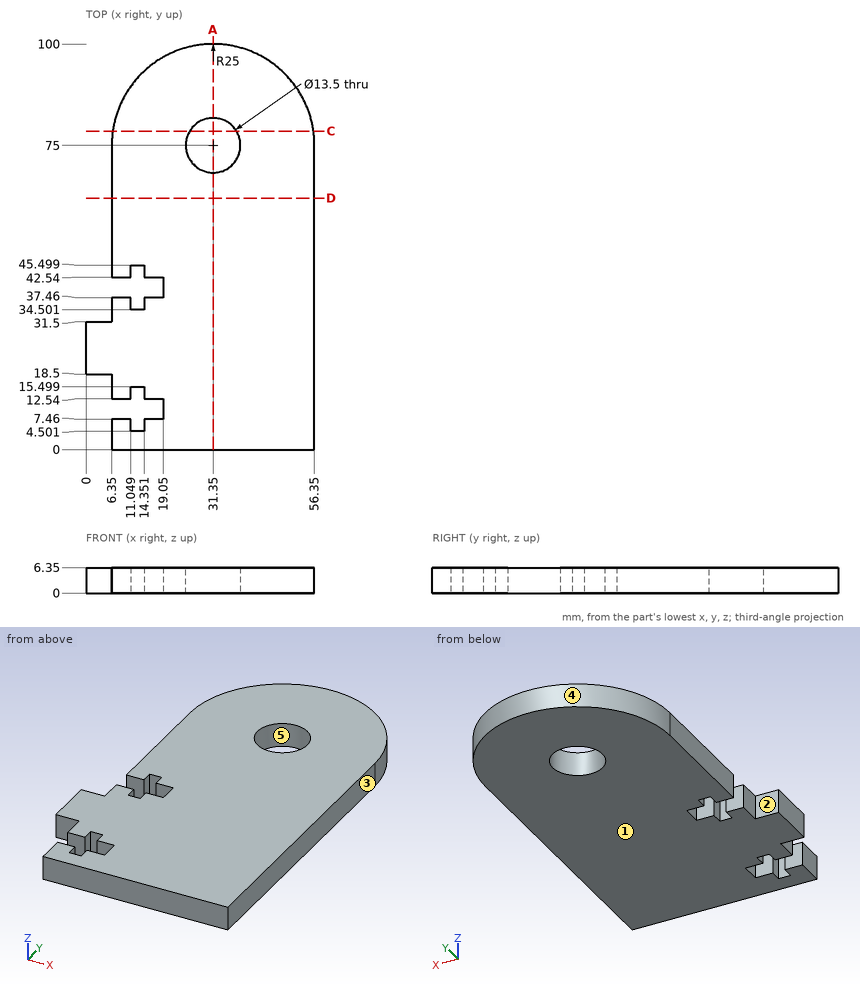
Can you work these out from the drawing? Everything is in mm from the part's minimum corner. A direction names the side the tool comes from. Round coordinates to 2 decimals unless told otherwise and drop trailing zeros. Loops run counter-clockwise (first coordinate to the right, second up) from the corner with the lowest first, then second, coordinate; pieces in that order, holes last. Notation, with made-up numbers: (81.25, 73) - (120.25, 73) arc R10 ccw to (120.25, 79) - close; hole circle Ø3 at (75, 62). An arc over 180 degrees is marked (long way). Answer as CSV lines item,"result".
1. We'd pull the mould along X, two halves only. Please class the marked faces 3, 4 and 5: +X half, -X half, draft (parallel to the pull), parting line (faces both ways), or undercut.
Filled in:
face 3,"+X half"
face 4,"parting line"
face 5,"undercut"
2. For pin 1 Ø1 at (x, z) = (13, 2) entering from +Y; pin 2 Ø3 at (x, z) = (4.5, 2) entering from +Y; pin 3 Ø1 at (x, z) = (13, 4.5) entering from -Y; pin 4 Ø1.8 at (y, z) = (33, 4.5) entering from -X, each with a flat end and sliding along its axis, tell me the tip position at first contact or that it passes through.
Filled in:
pin 1,"stops at y = 92.5"
pin 2,"stops at y = 31.5"
pin 3,"stops at y = 0"
pin 4,"stops at x = 6.35"
3. Please list where these lines run through material, in increasing order: line 1 along Y through (x, z) = (31.35, 1.75); line 2 along Y through (x, z) = (10, 2.5); line 3 along X through (y, z) = (47.5, 2.5). Write a range as [from, to].
Filled in:
line 1,"y = [0, 68.25], [81.75, 100]"
line 2,"y = [0, 7.46], [12.54, 37.46], [42.54, 88.01]"
line 3,"x = [6.35, 56.35]"
4. I want a section at A-A on x = 31.35. List the corners of the cut face in (y, z) for me, then the cut area to 3 significant figures.
Filled in:
outline,"(0, 0) - (68.25, 0) - (68.25, 6.35) - (0, 6.35) - close; (81.75, 0) - (100, 0) - (100, 6.35) - (81.75, 6.35) - close"
area,"549 mm^2"
5. I want a section at C-C on y = 78.5. List the corners of the cut face in (x, z) for me, then the cut area to 3 significant figures.
Filled in:
outline,"(6.6, 0) - (25.58, 0) - (25.58, 6.35) - (6.6, 6.35) - close; (37.12, 0) - (56.1, 0) - (56.1, 6.35) - (37.12, 6.35) - close"
area,"241 mm^2"
6. I want a section at D-D on y = 62. List the corners of the cut face in (x, z) for me, then the cut area to 4 significant figures.
Filled in:
outline,"(6.35, 0) - (56.35, 0) - (56.35, 6.35) - (6.35, 6.35) - close"
area,"317.5 mm^2"
7. On a 3-axis mill with a long thin cutter (end or side, diameter ignored), from which of +Z, -Z, +X, -X, +Y, -Y can I reach the whole of each face in a straight line? I mean the marked faces 1 and 2. Say none if no direction works.
Filled in:
face 1,"-Z, +X, -X, +Y, -Y"
face 2,"+Z, -Z, -X, +Y"
